```python
from build123d import *

# Parameters (mm, degrees)
SKETCH1_W           = 28
SKETCH1_H           = 95
BOSS_EXTRUDE1_DEPTH = 72
SKETCH2_W           = 13.730616592
SKETCH2_H           = 66.486096825
BOSS_EXTRUDE2_DEPTH = 20
SKETCH3_W           = 21.103215472
SKETCH3_H           = 11.539971669
SKETCH3_H_2         = 11.43433275
CUT_EXTRUDE1_DEPTH  = 65
SKETCH4_W           = 5.921037469
SKETCH4_H           = 7.955384718
CUT_EXTRUDE2_DEPTH  = 65


with BuildPart() as part:
    # Sketch1 → Boss-Extrude1 (new body)
    with BuildSketch(Plane(origin=(0, 0, 0), x_dir=(1, 0, 0), z_dir=(0, 1, 0))):
        with Locations((5.145873321, -3.829174664)):
            Rectangle(SKETCH1_W, SKETCH1_H)
    extrude(amount=BOSS_EXTRUDE1_DEPTH)

    # Sketch2 → Boss-Extrude2 (add)
    with BuildSketch(Plane(origin=(0, 72, 0), x_dir=(1, 0, 0), z_dir=(0, 1, 0))):
        with Locations((0.655068483, -2.824577048)):
            Rectangle(SKETCH2_W, SKETCH2_H)
    extrude(amount=BOSS_EXTRUDE2_DEPTH)

    # Sketch3 → Cut-Extrude1 (cut)
    with BuildSketch(Plane(origin=(0, 72, 0), x_dir=(1, 0, 0), z_dir=(0, 1, 0))):
        with Locations((1.697481057, -45.55918883)):
            Rectangle(SKETCH3_W, SKETCH3_H)
        with Locations((1.697481057, 37.953658961)):
            Rectangle(SKETCH3_W, SKETCH3_H_2)
    extrude(amount=-CUT_EXTRUDE1_DEPTH, mode=Mode.SUBTRACT)

    # Sketch4 → Cut-Extrude2 (cut)
    with BuildSketch(Plane(origin=(0, 7, 0), x_dir=(1, 0, 0), z_dir=(0, 1, 0))):
        with Locations((1.637392249, -47.351482305)):
            Rectangle(SKETCH4_W, SKETCH4_H)
        with Locations((1.637392249, 39.693132977)):
            Rectangle(SKETCH4_W, SKETCH4_H)
    extrude(amount=-CUT_EXTRUDE2_DEPTH, mode=Mode.SUBTRACT)


solid = part.part
```
CAD build for the part. Positions are in the model's coordinates, mm. A direction names the side the tool comes from. Coordinates: 2 decimals unless noted, no trailing zeros. Order: outer loops, then holes, each group sorted by start corner. A loop starts at its lowest first (then second) coordinate and runs counter-clockwise, first axis right, second up. Notation, with made-up numbers: (41, 11) - (56, 11) arc R15 cw to (56, 23) - close; hole circle Ø3 at (0, 27). An arc over 180 degrees is marked (long way). Answer in a Markdown table with one row per item.
1. Drill centre lines: L1, parallel to X at y = 87.5, z = 8; L2, parallel to Y at x = 12.5, z = 38; L3, parallel to X at y = 42.5, z = -36. Where is each one in solid material? Low to high. Write a range as from..to.
Answer:
| item | result |
|---|---|
| L1 | -6.21..7.52 |
| L2 | 0..72 |
| L3 | 12.25..19.15 |
2. Slice it at B-B, the plane y = 16. List the corners of the cut face in (x, z), then the cut area to 3 significant figures.
Answer:
| item | result |
|---|---|
| outline | (-8.85, -32.24) - (12.25, -32.24) - (12.25, -43.67) - (19.15, -43.67) - (19.15, 51.33) - (12.25, 51.33) - (12.25, 39.79) - (-8.85, 39.79) - close |
| area | 2,180 mm² |
3. Pull direction X, two halves, no side cores. Call faces 1 (the face through (-6.21, 82, 3)), 2 (the face through (1, 92, 2)), 3 (the face through (2, 4, -35.715)): +X half, -X half, draft (parallel to the pull), parting line (faces both ways), or undercut.
Answer:
| item | result |
|---|---|
| face 1 | -X half |
| face 2 | draft |
| face 3 | undercut |
4. Slice it at A-A, the plane z = -8.5. List the corners of the cut face in (x, y), then the cut area to 3 significant figures.
Answer:
| item | result |
|---|---|
| outline | (-8.85, 0) - (19.15, 0) - (19.15, 72) - (7.52, 72) - (7.52, 92) - (-6.21, 92) - (-6.21, 72) - (-8.85, 72) - close |
| area | 2,290 mm² |
5. Slice it at D-D, the plane x = 15.75. List the corners of the cut face in (y, z), then the cut area to 3 significant figures.
Answer:
| item | result |
|---|---|
| outline | (0, -43.67) - (72, -43.67) - (72, 51.33) - (0, 51.33) - close |
| area | 6,840 mm² |
6. 3-axis set-ups, long thin cutter, end or side, ignore diameter. For faces 4 (the face through (12.249, 40, -38)), 5 (the face through (4.598, 4, 47)), 6 (the face through (4.598, 4, -40)), 7 (the face through (1, 82, -30.418)), 8 (the face through (2, 7, 43)): which of +Z, -Z, +X, -X, +Y, -Y reach the whole face in a straight line?
Answer:
| item | result |
|---|---|
| face 4 | -Z, -X, +Y |
| face 5 | +Z, +Y, -Y |
| face 6 | -Z, +Y, -Y |
| face 7 | -Z, +X, -X, +Y |
| face 8 | +Z, -X, +Y |
7. Slice it at C-C, the plane x = -4.75. List the corners of the cut face in (y, z).
Answer:
| item | result |
|---|---|
| outline | (0, -43.67) - (7, -43.67) - (7, -32.24) - (72, -32.24) - (72, -30.42) - (92, -30.42) - (92, 36.07) - (72, 36.07) - (72, 39.79) - (7, 39.79) - (7, 51.33) - (0, 51.33) - close |
8. Flat gauge pins, fed straight in: P1, Ø11, axis at x = 1.5, y = 77, coming from the -Z side; P2, Ø3, axis at y = 76.5, z = 6, coming from the -X side; P3, Ø10, axis at y = 86, z = -1, coming from the +X side. Where does each tip first touch, or does it go through?
Answer:
| item | result |
|---|---|
| P1 | z = -32.24 |
| P2 | x = -6.21 |
| P3 | x = 7.52 |
